CAD build for the part. Positions are in the model's coordinates, mm. Coordinates: 2 decimals unless noted, no trailing zeros. Order: outer loops, then holes, each group sorted by start corner. A loop starts at its lowest first (then second) coordinate and runs counter-clockwise, first axis right, second up. Notation, with made-up numbers: (-32.5, -5) - (12.5, -5) arc R19 ccw to (12.5, -1) - close; hole circle Ø5 at (68, -31). An arc over 180 degrees is marked (long way). Return JSON: item names as keys, results as strings.
from build123d import *

# Parameters (mm, degrees)
CROQUIS1_W              = 100
CROQUIS1_H              = 139
CROQUIS1_R              = 3.5
CROQUIS1_R_2            = 2.65
CROQUIS1_R_3            = 2
SALIENTE_EXTRUIR1_DEPTH = 5
REDONDEO3_R             = 10


with BuildPart() as part:
    # Croquis1 → Saliente-Extruir1 (new body)
    with BuildSketch(Plane.XY):
        with Locations((50, 69.5)):
            Rectangle(CROQUIS1_W, CROQUIS1_H)
        with Locations((15, 115)):
            Circle(CROQUIS1_R, mode=Mode.SUBTRACT)
        with Locations((85, 115)):
            Circle(CROQUIS1_R, mode=Mode.SUBTRACT)
        with Locations((15, 55)):
            Circle(CROQUIS1_R_2, mode=Mode.SUBTRACT)
        with Locations((85, 55)):
            Circle(CROQUIS1_R_2, mode=Mode.SUBTRACT)
        with Locations((38, 131)):
            Circle(CROQUIS1_R_3, mode=Mode.SUBTRACT)
        with Locations((62, 131)):
            Circle(CROQUIS1_R_3, mode=Mode.SUBTRACT)
    extrude(amount=SALIENTE_EXTRUIR1_DEPTH)

    # Redondeo3
    redondeo3_edges = [part.edges().sort_by_distance(p)[0] for p in [
        (0, 139, 2.5),
        (100, 139, 2.5),
        (100, 0, 2.5),
        (0, 0, 2.5),
    ]]
    fillet(redondeo3_edges, radius=REDONDEO3_R)


solid = part.part
Item 1: Band-saw the part on D-D, the plane z = 3.95. List the corners of the cut face in (x, y), then the cut area to 3 significant figures.
Findings below:
{"outline": "(0, 10) arc R10 ccw to (10, 0) - (90, 0) arc R10 ccw to (100, 10) - (100, 129) arc R10 ccw to (90, 139) - (10, 139) arc R10 ccw to (0, 129) - close; hole circle Ø7 at (15, 115); hole circle Ø5.3 at (15, 55); hole circle Ø4 at (38, 131); hole circle Ø4 at (62, 131); hole circle Ø7 at (85, 115); hole circle Ø5.3 at (85, 55)", "area": "13,700 mm²"}
Item 2: Band-saw the part on C-C, the plane y = 115. List the corners of the cut face in (x, z).
Findings below:
{"outline": "(0, 0) - (11.5, 0) - (11.5, 5) - (0, 5) - close; (18.5, 0) - (81.5, 0) - (81.5, 5) - (18.5, 5) - close; (88.5, 0) - (100, 0) - (100, 5) - (88.5, 5) - close"}
Item 3: Band-saw the part on A-A, the plane x = 38. List the corners of the cut face in (y, z), then the cut area to 3 significant figures.
Findings below:
{"outline": "(0, 0) - (129, 0) - (129, 5) - (0, 5) - close; (133, 0) - (139, 0) - (139, 5) - (133, 5) - close", "area": "675 mm²"}
Item 4: Wall check: L1, parallel to Y at x = 15, z = 3.4; L2, parallel to X at y = 131, z = 3.7; L3, parallel to Y at x = 14, z = 4.15. Give the ranges that are in metal, low to high. Write a range as [from, to].
Findings below:
{"L1": "y = [0, 52.35], [57.65, 111.5], [118.5, 139]", "L2": "x = [0.2, 36], [40, 60], [64, 99.8]", "L3": "y = [0, 52.55], [57.45, 111.65], [118.35, 139]"}
Item 5: Drop a flat-ended pin along its axis: P1, Ø3.5, axis at x = 38, y = 131, coming from the +Z side. Give the stop position or say it passes through.
Findings below:
{"P1": "passes through"}
Item 6: Band-saw the part on B-B, the plane x = 15. List the corners of the cut face in (y, z).
Findings below:
{"outline": "(0, 0) - (52.35, 0) - (52.35, 5) - (0, 5) - close; (57.65, 0) - (111.5, 0) - (111.5, 5) - (57.65, 5) - close; (118.5, 0) - (139, 0) - (139, 5) - (118.5, 5) - close"}
Item 7: Mould opens along X. For faces 1 (the cylindrical face through (84.66, 57.63, 2.46)), 2 (the cylindrical face through (96.99, 136.15, 2.54)), 3 (the flat face through (49, 70, 0)) say: released by +X, released by -X, zero draft, split by the parting line, or undercut.
Findings below:
{"face 1": "undercut", "face 2": "released by +X", "face 3": "zero draft"}
